Part model, mm, in its own coordinate system. A direction names the side the tool comes from. Round coordinates to 2 decimals unless told otherwise and drop trailing zeros. Order: outer loops, then holes, each group sorted by start corner. A loop starts at its lowest first (then second) coordinate and runs counter-clockwise, first axis right, second up. Notation, with made-up numbers: (9.5, -9.5) - (63.5, -9.5) arc R22 cw to (63.5, 6.5) - close; hole circle Ø1 at (-19.5, -9.75). An arc over 180 degrees is marked (long way). Answer as a JSON object with one key per item and string values.
```python
from build123d import *

# Parameters (mm, degrees)
F0_R     = 11.176
F1_DEPTH = 5.715
F2_DEPTH = 5.715


# Not quite as in the source:
# - a feature names something its author has since deleted; it is built from what else it names


with BuildPart() as f1:
    # F0 (on Top) → F1 (new body)
    with BuildSketch(Plane.XY):
        with BuildLine():
            ThreePointArc((0, -15.24), (10.7763073453, -10.7763073453), (15.24, 0))
            ThreePointArc((15.24, 0), (10.7763073453, 10.7763073453), (0, 15.24))
            ThreePointArc((0, 15.24), (-10.7763073453, 10.7763073453), (-15.24, 0))
            ThreePointArc((-15.24, 0), (-10.7763073453, -10.7763073453), (0, -15.24))
        make_face()
        Circle(F0_R, mode=Mode.SUBTRACT)
        with BuildLine():
            Line((27.94, 0), (15.24, 0))
            ThreePointArc((15.24, 0), (10.7763073453, -10.7763073453), (0, -15.24))
            Line((0, -15.24), (40.64, -15.24))
            Line((40.64, -15.24), (40.64, 0))
            Line((40.64, 0), (27.94, 0))
        make_face()
        with BuildLine():
            ThreePointArc((0, 15.24), (10.7763073453, 10.7763073453), (15.24, 0))
            Line((15.24, 0), (15.24, 40.64))
            Line((15.24, 40.64), (0, 40.64))
            Line((0, 40.64), (0, 27.94))
            Line((0, 27.94), (0, 15.24))
        make_face()
        with BuildLine():
            ThreePointArc((-15.24, 0), (-10.7763073453, 10.7763073453), (0, 15.24))
            Line((0, 15.24), (-40.64, 15.24))
            Line((-40.64, 15.24), (-40.64, 0))
            Line((-40.64, 0), (-27.94, 0))
            Line((-27.94, 0), (-15.24, 0))
        make_face()
        with BuildLine():
            Line((0, -27.94), (0, -15.24))
            ThreePointArc((0, -15.24), (-10.7763073453, -10.7763073453), (-15.24, 0))
            Line((-15.24, 0), (-15.24, -40.64))
            Line((-15.24, -40.64), (0, -40.64))
            Line((0, -40.64), (0, -27.94))
        make_face()
    extrude(amount=F1_DEPTH)

    # F0 (on Top) → F2 (join)
    with BuildSketch(Plane.XY):
        with BuildLine():
            ThreePointArc((0, -15.24), (10.7763073453, -10.7763073453), (15.24, 0))
            ThreePointArc((15.24, 0), (10.7763073453, 10.7763073453), (0, 15.24))
            ThreePointArc((0, 15.24), (-10.7763073453, 10.7763073453), (-15.24, 0))
            ThreePointArc((-15.24, 0), (-10.7763073453, -10.7763073453), (0, -15.24))
        make_face()
        Circle(F0_R, mode=Mode.SUBTRACT)
        with BuildLine():
            Line((27.94, 0), (15.24, 0))
            ThreePointArc((15.24, 0), (10.7763073453, -10.7763073453), (0, -15.24))
            Line((0, -15.24), (40.64, -15.24))
            Line((40.64, -15.24), (40.64, 0))
            Line((40.64, 0), (27.94, 0))
        make_face()
        with BuildLine():
            ThreePointArc((0, 15.24), (10.7763073453, 10.7763073453), (15.24, 0))
            Line((15.24, 0), (15.24, 40.64))
            Line((15.24, 40.64), (0, 40.64))
            Line((0, 40.64), (0, 27.94))
            Line((0, 27.94), (0, 15.24))
        make_face()
        with BuildLine():
            ThreePointArc((-15.24, 0), (-10.7763073453, 10.7763073453), (0, 15.24))
            Line((0, 15.24), (-40.64, 15.24))
            Line((-40.64, 15.24), (-40.64, 0))
            Line((-40.64, 0), (-27.94, 0))
            Line((-27.94, 0), (-15.24, 0))
        make_face()
        with BuildLine():
            Line((0, -27.94), (0, -15.24))
            ThreePointArc((0, -15.24), (-10.7763073453, -10.7763073453), (-15.24, 0))
            Line((-15.24, 0), (-15.24, -40.64))
            Line((-15.24, -40.64), (0, -40.64))
            Line((0, -40.64), (0, -27.94))
        make_face()
        Polygon((27.94, 15.24), (27.94, 0), (40.64, 0), align=None)
        Polygon((-15.24, 27.94), (0, 27.94), (0, 40.64), align=None)
        Polygon((15.24, -27.94), (0, -27.94), (0, -40.64), align=None)
        Polygon((-27.94, -15.24), (-27.94, 0), (-40.64, 0), align=None)
    extrude(amount=F2_DEPTH)


solid = f1.part
```
Item 1: Two-plate mould, pull along Y, no slides. Class faces 4 (the flat face through (-20, 15.24, 3)), 5 (the flat face through (8, 40.64, 3)), 6 (the cylindrical face through (-8.87, -6.8, 2.82)), 7 (the flat face through (-27.94, -8, 3)): pulls with the +Y half, pulls with the -Y half, needs draft (parallel to the pull), parting line crosses it, or undercut.
Taken from the geometry:
{"face 4": "undercut", "face 5": "pulls with the +Y half", "face 6": "undercut", "face 7": "needs draft"}
Item 2: Drop flat-ended pins along their axis: P1, Ø3, axis at x = -15.5, z = 3, coming from the +Y side; P2, Ø3, axis at x = -21.5, z = 4, coming from the -Y side; P3, Ø1.7, axis at y = -19.5, z = 3.5, coming from the +X side. Give the stop position or say it passes through.
Taken from the geometry:
{"P1": "y = 28.97", "P2": "y = 0", "P3": "x = 0"}
Item 3: Probe L1, parallel to X at y = 1.5, z = 1.6; L2, parallel to Y at x = 2, z = 3.65; L3, parallel to Y at x = -27, z = 0.45. List the from-to ranges inside material, lowest first. Write a range as from..to.
Taken from the geometry:
{"L1": "-40.64..-11.07, 11.07..15.24, 27.94..39.39", "L2": "-38.97..-27.94, -15.24..-11, 11..40.64", "L3": "0..15.24"}
Item 4: Cut at B-B (y = 9). Write the cut outline in (x, z) (3 decimals).
Taken from the geometry:
{"outline": "(-40.64, 0) - (-6.626, 0) - (-6.626, 5.715) - (-40.64, 5.715) - close; (6.626, 0) - (15.24, 0) - (15.24, 5.715) - (6.626, 5.715) - close; (27.94, 0) - (33.14, 0) - (33.14, 5.715) - (27.94, 5.715) - close"}
Item 5: Tool access for faces 1 (the flat face through (-15.24, -20, 3)), 2 (the flat face through (-8, 27.94, 3)), 3 (the flat face through (8, -27.94, 3)): list every direction of +Z, -Z, +X, -X, +Y, -Y with a clear straight run to the whole face (end or side of a thin tool).
Taken from the geometry:
{"face 1": "+Z, -Z, -Y", "face 2": "+Z, -Z, -X", "face 3": "+Z, -Z, +X"}
Item 6: Cut at D-D (x = 16.5). Write the cut outline in (y, z) (3 decimals).
Taken from the geometry:
{"outline": "(-15.24, 0) - (0, 0) - (0, 5.715) - (-15.24, 5.715) - close"}
Item 7: Cut at A-A (z = 1). Write the cut outline in (x, y).
Taken from the geometry:
{"outline": "(-40.64, 0) - (-27.94, -15.24) - (-27.94, 0) - (-15.24, 0) - (-15.24, -40.64) - (0, -40.64) - (15.24, -27.94) - (0, -27.94) - (0, -15.24) - (40.64, -15.24) - (40.64, 0) - (27.94, 15.24) - (27.94, 0) - (15.24, 0) - (15.24, 40.64) - (0, 40.64) - (-15.24, 27.94) - (0, 27.94) - (0, 15.24) - (-40.64, 15.24) - close; hole circle Ø22.35 at (0, 0)"}
Item 8: Cut at C-C (x = -13). Write the cut outline in (y, z) (3 decimals).
Taken from the geometry:
{"outline": "(-40.64, 0) - (15.24, 0) - (15.24, 5.715) - (-40.64, 5.715) - close; (27.94, 0) - (29.807, 0) - (29.807, 5.715) - (27.94, 5.715) - close"}
